Input: part model. Units: mm. Frame: model coordinates. Face numbers are marked on the shaded views. A direction names the side the tool comes from. Round coordinates to 2 decimals unless told otherwise and drop trailing zeros. Order: outer loops, then holes, each group sorted by start corner. A loop starts at its lowest first (then second) coordinate and runs counter-clockwise, first axis right, second up.
Item 1: Cut plane B-B on x = 38.5. Output: boundary loops of the cut face in (y, z).
Item 2: Cut plane A-A on z = 24.6. Output: boundary loops of the cut face in (x, y), then the cut area to 3 significant figures.
Item 3: Line query: L1, parallel to Z at x = 22.5, y = 4.95; L2, parallel to Y at x = -25, z = 32; L3, parallel to Y at x = -38, z = 1. Output: solid intervals per line, ascending.
Item 4: Reachability of the marked faces 1 and 2 from +Z, -Z, +X, -X, +Y, -Y: full face, straight path, thin tool, end or side. Return the list, or none.
Item 5: Cut plane D-D on z = 31. Output: boundary loops of the cut face in (x, y), then the cut area to 3 significant figures.
Item 6: First-contact query: pin 1 (3 mm diameter, centred on x = 32, z = 24, fed in from -Y); pin 2 (5 mm diameter, centred on x = 38.5, y = 0, fed in from -Z); pin 3 (0.8 mm diameter, centred on y = 5.5, z = 13, fed in from -X); pin 4 (1.6 mm diameter, centred on y = 5, z = 17.5, fed in from +X). Flat tips, straight axial feed; report the tip coordinate or a pass-through.
Item 7: Cut plane C-C on y = -1.25. Output: boundary loops of the cut face in (x, z), then the cut area to 3 significant figures.
Autodesk Inventor part; units mm, degrees
ref_plane "YZ Plane" through (0, 0, 0) normal (1, 0, 0) x (0, 1, 0)
ref_plane "XZ Plane" through (0, 0, 0) normal (0, 1, 0) x (-1, 0, 0)
ref_plane "XY Plane" through (0, 0, 0) normal (0, 0, 1) x (1, 0, 0)
sketch "Sketch1" plane through (0, 0, 0) normal (0, 0, 1) x (1, 0, 0)
  line L0 (-35.5, 4.5) -> (35.5, 4.5)
  line L1 (35.5, 4.5) -> (35.5, -4.5)
  line L2 (35.5, -4.5) -> (-35.5, -4.5)
  line L3 (-35.5, -4.5) -> (-35.5, 4.5)
  line L4 (-35.5, 4.5) -> (-41.5, 4.5)
  line L5 (-41.5, 4.5) -> (-41.5, -4.5)
  line L6 (-41.5, -4.5) -> (-35.5, -4.5)
  line L7 (-35.5, -4.5) -> (-35.5, 4.5)
  line L8 (35.5, 4.5) -> (41.5, 4.5)
  line L9 (41.5, 4.5) -> (41.5, -4.5)
  line L10 (41.5, -4.5) -> (35.5, -4.5)
  line L11 (35.5, -4.5) -> (35.5, 4.5)
  line L12 (-41.5, 0) -> (41.5, 0) construction
  circle A0 centre (-38.5, 0) radius 2.25
  circle A1 centre (38.5, 0) radius 2.25
  line L13 (0, 4.5) -> (0, -4.5) construction
  line L14 (-32.5, 4.5) -> (32.5, 4.5)
  line L15 (32.5, 4.5) -> (32.5, 6)
  line L16 (32.5, 6) -> (-32.5, 6)
  line L17 (-32.5, 6) -> (-32.5, 4.5)
  line L18 (-32.5, 6) -> (-41.5, 6)
  line L19 (-41.5, 6) -> (-41.5, 4.5)
  line L20 (-41.5, 4.5) -> (-32.5, 4.5)
  line L21 (-32.5, 4.5) -> (-32.5, 6)
  line L22 (32.5, 6) -> (41.5, 6)
  line L23 (41.5, 6) -> (41.5, 4.5)
  line L24 (41.5, 4.5) -> (32.5, 4.5)
  line L25 (32.5, 4.5) -> (32.5, 6)
  point P0 (0, 0)
  point P1 (0, 0)
  point P2 (0, 7)
  point P3 (0, 0)
  point P4 (0, 6)
  dimension "d0" = 9
  dimension "d1" = 71
  dimension "d2" = 4.5
  dimension "d3" = 4.5
  dimension "d4" = 3
  dimension "d5" = 3
  dimension "d6" = 3
  dimension "d7" = 3
  dimension "d12" = 65
  dimension "d13" = 1.5
extrude "Extrusion1" add sketch "Sketch1" along normal blind 1.5
extrude "Extrusion2" add sketch "Sketch1" along normal blind 40 contours L17 L16 L15 L0
sketch "Sketch2" plane through (-41.5, 4.5, 1.5) normal (0, -1, 0) x (1, 0, 0)
  line L0 (74, 0) -> (74, 38.5)
  line L1 (9, 38.5) -> (74, 38.5)
  line L2 (9, 0) -> (9, 38.5)
  circle A0 centre (19, 23.1) radius 5.5
  circle A1 centre (64, 23.1) radius 5.5
  line L3 (41.5, 38.5) -> (41.5, -1.5) construction
  line L4 (30.1, 33.5) -> (52.9, 33.5)
  line L5 (52.9, 33.5) -> (52.9, 12.7)
  line L6 (52.9, 12.7) -> (30.1, 12.7)
  line L7 (30.1, 12.7) -> (30.1, 33.5)
  line L8 (30.1, 23.1) -> (52.9, 23.1) construction
  point P0 (41.5, 33.5)
  dimension "d16" = 11
  dimension "d17" = 11
  dimension "d19" = 10
  dimension "d21" = 10
  dimension "d22" = 5
  dimension "d23" = 22.8
  dimension "d24" = 20.8
extrude "Extrusion3" cut sketch "Sketch2" against normal blind 10
fillet "Fillet1" radius 10 2 edges at (-32.5, 5.25, 40) (32.5, 5.25, 40)
properties part number "MotorBar"
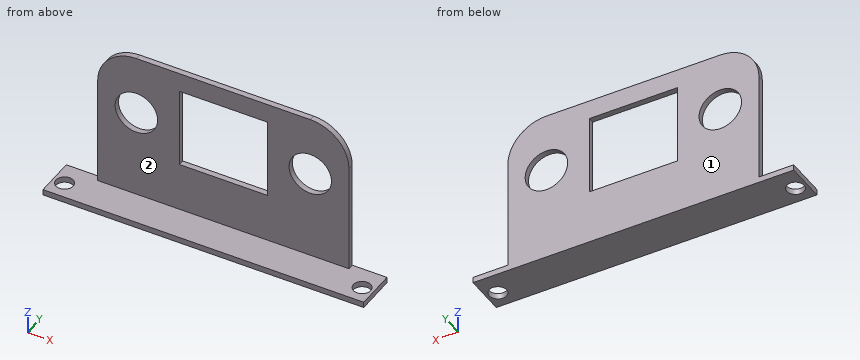
From the geometry:
1. outline: (-4.5, 0) - (-2.25, 0) - (-2.25, 1.5) - (-4.5, 1.5) - close; (2.25, 0) - (6, 0) - (6, 1.5) - (2.25, 1.5) - close
2. outline: (-32.5, 4.5) - (-28, 4.5) - (-28, 6) - (-32.5, 6) - close; (-17, 4.5) - (-11.4, 4.5) - (-11.4, 6) - (-17, 6) - close; (11.4, 4.5) - (17, 4.5) - (17, 6) - (11.4, 6) - close; (28, 4.5) - (32.5, 4.5) - (32.5, 6) - (28, 6) - close
2. area: 30.3 mm2
3. L1: z = 0 to 19.1, 30.1 to 40
3. L2: y = 4.5 to 6
3. L3: y = -4.5 to -2.19, 2.19 to 6
4. face 1: +Z, -Z, +X, -X, +Y
4. face 2: +Z, +X, -X, -Y
5. outline: (-32.45, 4.5) - (-11.4, 4.5) - (-11.4, 6) - (-32.45, 6) - close; (11.4, 4.5) - (32.45, 4.5) - (32.45, 6) - (11.4, 6) - close
5. area: 63.1 mm2
6. pin 1: stops at y = 4.5
6. pin 2: stops at z = 0
6. pin 3: stops at x = -32.5
6. pin 4: stops at x = 32.5
7. outline: (-41.5, 0) - (-40.37, 0) - (-40.37, 1.5) - (-41.5, 1.5) - close; (-36.63, 0) - (36.63, 0) - (36.63, 1.5) - (-36.63, 1.5) - close; (40.37, 0) - (41.5, 0) - (41.5, 1.5) - (40.37, 1.5) - close
7. area: 113 mm2
